from build123d import *

# Parameters (mm, degrees)
F0_R     = 11
F1_DEPTH = 3
F3_DEPTH = 10
F4_SIZE  = 0.5


# Not quite as in the source:
# - a fillet or chamfer that OpenCascade refuses, or shapes differently, is made with other operations: its cross-section is extruded or revolved along the edge and cut away or added


with BuildPart() as f1:
    # F0 (on Top) → F1 (new body)
    with BuildSketch(Plane.XY):
        Circle(F0_R)
    extrude(amount=F1_DEPTH)

    # F2 (on face) → F3 (join)
    with BuildSketch(Plane.XY.offset(3)):
        Polygon((0.8564302523, -3.5647384976), (3.5153692229, -1.0406788937), (2.6589389706, 2.5240596039), (-0.8564302523, 3.5647384976), (-3.5153692229, 1.0406788937), (-2.6589389706, -2.5240596039), align=None)
    extrude(amount=F3_DEPTH)

    # F4
    f4_edges = [f1.edges().sort_by_distance(p)[0] for p in [
        (2.1859, -2.302709, 13),
        (3.087154, 0.74169, 13),
        (0.901254, 3.044399, 13),
        (-2.1859, 2.302709, 13),
        (-3.087154, -0.74169, 13),
        (-0.901254, -3.044399, 13),
    ]]
    chamfer(f4_edges, length=F4_SIZE)

    # F5: fillet of radius 5 on 1 edges, made by hand

    # F5_s1 → F5_t2 (revolve, cut)
    with BuildSketch(Plane.XZ):
        with BuildLine():
            ThreePointArc((6.417424305, 3), (9.1560370926, 2.1833001327), (11, 0))
            Line((11, 0), (11, 3))
            Line((11, 3), (6.417424305, 3))
        make_face()
    revolve(axis=Axis((0, 0, 3), (0, 0, 1)), mode=Mode.SUBTRACT)


solid = f1.part
Read the model definition and answer for the solid it produces. Units are mm, in the model's axes. A direction names the side the tool comes from. Give positions to 0.01 mm unless a question says otherwise; leave off trailing zeros. Loops run counter-clockwise (first coordinate to the right, second up) from the corner with the lowest first, then second, coordinate; pieces in that order, holes last. Notation, with made-up numbers: (-9.75, 8) -> (-1.75, 8) arc R12 ccw to (-1.75, 27) -> close; hole circle Ø3 at (-26, 80). An arc over 180 degrees is marked (long way). Use a Markdown table: item, result.
Q1. Section B-B, the plane z = 1.5 is taken. Determine the outline of the cut face in (x, y).
Solved:
| item | result |
|---|---|
| outline | circle Ø19.98 at (0, 0) |
Q2. Find the intervals of material crossed by line 1 along Z through (x, y) = (4.5, -5); line 2 along Z through (x, y) = (0, 8); line 3 along Y through (x, z) = (-1, 12), in increasing order.
Solved:
| item | result |
|---|---|
| line 1 | z = 0 to 2.99 |
| line 2 | z = 0 to 2.74 |
| line 3 | y = -3.02 to 3.43 |
Q3. Each of these flat-tipped pins is pushed along its axis until it touches: pin 1 (3 mm diameter, centred on x = 7, y = -7.5, fed in from -Z); pin 2 (6 mm diameter, centred on x = -8.5, z = 7.5, fed in from +Y); pin 3 (6 mm diameter, centred on y = -6, z = 2.5, fed in from -X); pin 4 (1.5 mm diameter, centred on x = -3.5, z = 7.5, fed in from +Y). Where does it stop, or does it pass through?
Solved:
| item | result |
|---|---|
| pin 1 | stops at z = 0 |
| pin 2 | passes through |
| pin 3 | stops at x = -10.12 |
| pin 4 | stops at y = 1.77 |
Q4. Section A-A, the plane z = 8.5 is taken. Determine the outline of the cut face in (x, y), then the cut area to 3 significant figures.
Solved:
| item | result |
|---|---|
| outline | (-3.52, 1.04) -> (-2.66, -2.52) -> (0.86, -3.56) -> (3.52, -1.04) -> (2.66, 2.52) -> (-0.86, 3.56) -> close |
| area | 34.9 mm^2 |
Q5. A tool of negligible diameter and unlimited length cuts with its end or side. For faces 1 (the face through (-0.926, -3.037, 7.684)), 2 (the face through (0.926, 3.037, 7.684)), 3 (the face through (-2.17, 2.32, 7.68)), 4 (the face through (2.17, -2.32, 7.68)), 5 (the face through (-2, 3, 3)), from which of +Z, -Z, +X, -X, +Y, -Y can it reach the whole face along a straight path? Write none if from no direction.
Solved:
| item | result |
|---|---|
| face 1 | +Z, -X, -Y |
| face 2 | +Z, +X, +Y |
| face 3 | +Z, -X, +Y |
| face 4 | +Z, +X, -Y |
| face 5 | +Z |
